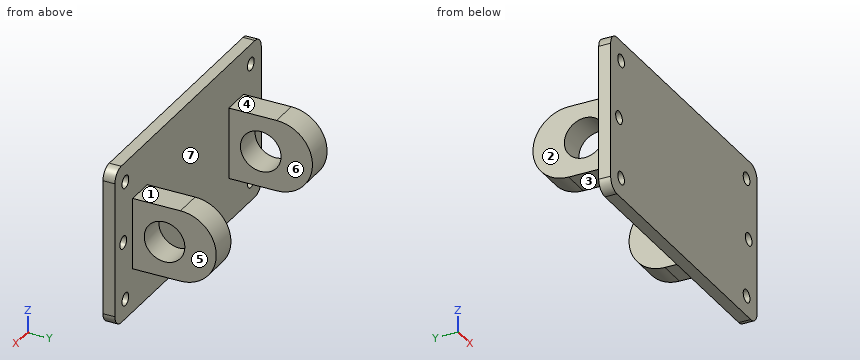
```python
from build123d import *

# Parameters (mm, degrees)
EXTRUDE_1_DEPTH     = 3
SKETCH_2_W          = 7
SKETCH_2_H          = 18
EXTRUDE_2_DEPTH     = 12
SKETCH_3_R          = 9
EXTRUDE_3_DEPTH     = 7
EXTRUDE_START       = -7
SKETCH_4_R          = 9
EXTRUDE_4_DEPTH     = 7
SKETCH_5_R          = 5
CUT_EXTRUDE_1_DEPTH = 69.980069585
SKETCH_6_R          = 1.6
CUT_EXTRUDE_2_DEPTH = 46.453272709
SKETCH_7_R          = 1.6
CUT_EXTRUDE_3_DEPTH = 10
SKETCH_8_R          = 5.1
CUT_EXTRUDE_4_DEPTH = 69.980069585


with BuildPart() as part:
    # 草图1 → 凸台-拉伸1 (new body)
    with BuildSketch(Plane(origin=(0, 0, 0), x_dir=(1, 0, 0), z_dir=(0, 1, 0))):
        with BuildLine():
            Line((-32, -20), (32, -20))
            ThreePointArc((32, -20), (34.121320344, -19.121320344), (35, -17))
            Line((35, -17), (35, 17))
            ThreePointArc((35, 17), (34.121320344, 19.121320344), (32, 20))
            Line((32, 20), (-32, 20))
            ThreePointArc((-32, 20), (-34.121320344, 19.121320344), (-35, 17))
            Line((-35, 17), (-35, -17))
            ThreePointArc((-35, -17), (-34.121320344, -19.121320344), (-32, -20))
        make_face()
    extrude(amount=EXTRUDE_1_DEPTH)

    # 草图2 → 凸台-拉伸2 (add)
    with BuildSketch(Plane(origin=(0, 3, 0), x_dir=(1, 0, 0), z_dir=(0, 1, 0))):
        with Locations((23, 0)):
            Rectangle(SKETCH_2_W, SKETCH_2_H)
    extrude_2 = extrude(amount=EXTRUDE_2_DEPTH)

    # 镜向1: 凸台-拉伸2 across plane
    add(extrude_2.mirror(Plane(origin=(0, 0, 0), x_dir=(0, 0, 1), z_dir=(1, 0, 0))))

    # 草图3 → 凸台-拉伸3 (add)
    with BuildSketch(Plane(origin=(26.5, 0, 0), x_dir=(0, 0, -1), z_dir=(1, 0, 0))):
        with Locations((0, 15)):
            Circle(SKETCH_3_R)
    extrude(amount=-EXTRUDE_3_DEPTH)

    # 草图4 → 凸台-拉伸4 (add)
    with BuildSketch(Plane.ZY.offset(26.5).offset(EXTRUDE_START)):
        with Locations((0, 15)):
            Circle(SKETCH_4_R)
    extrude(amount=EXTRUDE_4_DEPTH)

    # 草图5 → 切除-拉伸1 (cut, through all)
    with BuildSketch(Plane(origin=(26.5, 0, 0), x_dir=(0, 0, -1), z_dir=(1, 0, 0))):
        with Locations((0, 11)):
            Circle(SKETCH_5_R)
    extrude(amount=-CUT_EXTRUDE_1_DEPTH, mode=Mode.SUBTRACT)

    # 草图6 → 切除-拉伸2 (cut, through all)
    with BuildSketch(Plane(origin=(0, 3, 0), x_dir=(1, 0, 0), z_dir=(0, 1, 0))):
        with Locations(Location((-31, 0, 0), (0, 0, 270))):
            Circle(SKETCH_6_R)
        with Locations(Location((31, 0, 0), (0, 0, 270))):
            Circle(SKETCH_6_R)
    extrude(amount=-CUT_EXTRUDE_2_DEPTH, mode=Mode.SUBTRACT)

    # 草图7 → 切除-拉伸3 (cut)
    with BuildSketch(Plane(origin=(0, 3, 0), x_dir=(1, 0, 0), z_dir=(0, 1, 0))):
        with Locations(Location((-30, 15, 0), (0, 0, 270))):
            Circle(SKETCH_7_R)
        with Locations(Location((30, 15, 0), (0, 0, 270))):
            Circle(SKETCH_7_R)
        with Locations(Location((30, -15, 0), (0, 0, 270))):
            Circle(SKETCH_7_R)
        with Locations(Location((-30, -15, 0), (0, 0, 270))):
            Circle(SKETCH_7_R)
    extrude(amount=-CUT_EXTRUDE_3_DEPTH, mode=Mode.SUBTRACT)

    # 草图8 → 切除-拉伸4 (cut, through all)
    with BuildSketch(Plane(origin=(26.5, 0, 0), x_dir=(0, 0, -1), z_dir=(1, 0, 0))):
        with Locations((0, 11)):
            Circle(SKETCH_8_R)
    extrude(amount=-CUT_EXTRUDE_4_DEPTH, mode=Mode.SUBTRACT)


solid = part.part
```
The model under review builds one solid part; all positions refer to its coordinate system, in mm. Face numbers are marked on the shaded views. A direction names the side the tool comes from. Give positions to 0.01 mm unless a question says otherwise; leave off trailing zeros. Write each loop counter-clockwise with the first axis right and the second up, starting at its lowest first coordinate (ties: lowest second). Pieces come first, ordered by that corner, then holes.
(1) Consider section B-B, the plane y = 11. Give the boundary of the cut face in (x, z), and give its area (3 significant figures).
(2) The part is to be moulded in two halves that separate along X. For the marked faces 4, 5, 6 and 7, say which applies: released by +X, released by -X, zero draft, split by the parting line, or undercut.
(3) Tool access review of the marked faces 1, 2 and 3: name each direction out of +Z, -Z, +X, -X, +Y, -Y from which nothing blocks a thin tool from reaching the whole face with its end or side.
(4) Consider section D-D, the plane x = 11.5. Give the boundary of the cut face in (y, z).
(5) Consider section A-A, the plane z = 0. Give the boundary of the cut face in (x, y), and give its area (3 significant figures).
(6) For P1, Ø5, axis at x = -30, z = -15, coming from the -Y side; P2, Ø3.5, axis at x = 23.5, y = 7.5, coming from the -Z side; P3, Ø5.5, axis at y = 18, z = 1.5, coming from the +X side; P4, Ø9, axis at y = 11.5, z = -0.5, coming from the -X side, all flat-tipped, find the tip position at first contact; note any pin that passes through.
(7) Consider section C-C, the plane y = 19.5. Give the boundary of the cut face in (x, z), and give its area (3 significant figures).
(8) To check wall thickness, follow L1, parallel to X at y = 0.9, z = -15; L2, parallel to X at y = 1.2, z = 0; L3, parallel to Y at x = -24, z = 0. State the ranges of each line that lie inside material, in increasing order.
Returned:
1. outline: (-26.5, -9) - (-19.5, -9) - (-19.5, -5.1) - (-26.5, -5.1) - close; (-26.5, 5.1) - (-19.5, 5.1) - (-19.5, 9) - (-26.5, 9) - close; (19.5, -9) - (26.5, -9) - (26.5, -5.1) - (19.5, -5.1) - close; (19.5, 5.1) - (26.5, 5.1) - (26.5, 9) - (19.5, 9) - close
1. area: 109 mm2
2. face 4: zero draft
2. face 5: released by +X
2. face 6: undercut
2. face 7: undercut
3. face 1: +Z, +X, -X, +Y
3. face 2: +Z, -Z, -X, +Y
3. face 3: -Z, +X, -X, +Y
4. outline: (0, -20) - (3, -20) - (3, 20) - (0, 20) - close
5. outline: (-35, 0) - (-32.6, 0) - (-32.6, 3) - (-35, 3) - close; (-29.4, 0) - (29.4, 0) - (29.4, 3) - (26.5, 3) - (26.5, 5.9) - (19.5, 5.9) - (19.5, 3) - (-19.5, 3) - (-19.5, 5.9) - (-26.5, 5.9) - (-26.5, 3) - (-29.4, 3) - close; (-26.5, 16.1) - (-19.5, 16.1) - (-19.5, 24) - (-26.5, 24) - close; (19.5, 16.1) - (26.5, 16.1) - (26.5, 24) - (19.5, 24) - close; (32.6, 0) - (35, 0) - (35, 3) - (32.6, 3) - close
5. area: 342 mm2
6. P1: stops at y = 0
6. P2: stops at z = -9
6. P3: stops at x = 26.5
6. P4: stops at x = -26.5
7. outline: (-26.5, -7.79) - (-19.5, -7.79) - (-19.5, 7.79) - (-26.5, 7.79) - close; (19.5, -7.79) - (26.5, -7.79) - (26.5, 7.79) - (19.5, 7.79) - close
7. area: 218 mm2
8. L1: x = -35 to -31.6, -28.4 to 28.4, 31.6 to 35
8. L2: x = -35 to -32.6, -29.4 to 29.4, 32.6 to 35
8. L3: y = 0 to 5.9, 16.1 to 24
